Design review of the part built by this model. Coordinates are the model's own, in mm. Face numbers are marked on the shaded views. A direction names the side the tool comes from. Give positions to 0.01 mm unless a question says otherwise; leave off trailing zeros. Write each loop counter-clockwise with the first axis right and the second up, starting at its lowest first coordinate (ties: lowest second). Pieces come first, ordered by that corner, then holes. Notation, with made-up numbers: M 47.5,86 L 80.5,86 A17 cw 80.5,112 Z; hole C 20.5,68.5 d10. An arc over 180 degrees is marked long. Use one line per item in the form item = value. Start each with the question number.
from build123d import *

# Parameters (mm, degrees)
SKETCH1_R               = 25
BOSS_EXTRUDE1_DEPTH     = 10
SKETCH1_3_R             = 12.5
SKETCH1_3_R_2           = 6
BOSS_EXTRUDE2_DEPTH     = 35
CUT_EXTRUDE1_START      = 5
CUT_EXTRUDE1_DEPTH      = 5
CUT_EXTRUDE2_DEPTH      = 50.749371855
CUT_EXTRUDE2_DEPTH_BACK = 50.749371855
SKETCH3_R               = 2.5
CUT_EXTRUDE3_DEPTH      = 50.749371926
CIRPATTERN1_COUNT       = 6
CHAMFER1_SIZE           = 5


with BuildPart() as part:
    # Sketch1 → Boss-Extrude1 (new body)
    with BuildSketch(Plane(origin=(0, 0, 0), x_dir=(1, 0, 0), z_dir=(0, 1, 0))):
        with Locations(Location((0, 0, 0), (0, 0, 270))):
            Circle(SKETCH1_R)
    extrude(amount=BOSS_EXTRUDE1_DEPTH)

    # Sketch1<3> → Boss-Extrude2 (add)
    with BuildSketch(Plane(origin=(0, 0, 0), x_dir=(1, 0, 0), z_dir=(0, 1, 0))):
        with Locations(Location((0, 0, 0), (0, 0, 270))):
            Circle(SKETCH1_3_R)
        with Locations(Location((0, 0, 0), (0, 0, 270))):
            Circle(SKETCH1_3_R_2, mode=Mode.SUBTRACT)
    extrude(amount=BOSS_EXTRUDE2_DEPTH)

    # Sketch1<5> → Cut-Extrude1 (cut)
    with BuildSketch(Plane(origin=(0, 0, 0), x_dir=(1, 0, 0), z_dir=(0, 1, 0)).offset(CUT_EXTRUDE1_START)):
        with BuildLine():
            ThreePointArc((20, 15), (0, 25), (-20, 15))
            Line((-20, 15), (20, 15))
        make_face()
    extrude(amount=CUT_EXTRUDE1_DEPTH, mode=Mode.SUBTRACT)

    # Sketch2 → Cut-Extrude2 (cut, two sides: drawn at the far end of the back side and taken through both)
    with BuildSketch(Plane.XY.offset(-CUT_EXTRUDE2_DEPTH_BACK)):
        with BuildLine():
            Line((0, 25.5), (0, 35))
            Line((0, 35), (-2.5, 35))
            Line((-2.5, 35), (-2.5, 23))
            ThreePointArc((-2.5, 23), (-1.767766953, 24.767766953), (0, 25.5))
        make_face()
        with BuildLine():
            Line((2.5, 35), (0, 35))
            Line((0, 35), (0, 25.5))
            ThreePointArc((0, 25.5), (1.767766953, 24.767766953), (2.5, 23))
            Line((2.5, 23), (2.5, 35))
        make_face()
        with BuildLine():
            ThreePointArc((2.5, 23), (1.767766953, 24.767766953), (0, 25.5))
            Line((0, 25.5), (0, 23))
            Line((0, 23), (2.5, 23))
        make_face()
        with BuildLine():
            Line((0, 23), (0, 25.5))
            ThreePointArc((0, 25.5), (-1.767766953, 24.767766953), (-2.5, 23))
            Line((-2.5, 23), (0, 23))
        make_face()
        with BuildLine():
            Line((2.5, 23), (0, 23))
            Line((0, 23), (0, 20.5))
            ThreePointArc((0, 20.5), (1.767766953, 21.232233047), (2.5, 23))
        make_face()
        with BuildLine():
            Line((0, 20.5), (0, 23))
            Line((0, 23), (-2.5, 23))
            ThreePointArc((-2.5, 23), (-1.767766953, 21.232233047), (0, 20.5))
        make_face()
    extrude(amount=CUT_EXTRUDE2_DEPTH + CUT_EXTRUDE2_DEPTH_BACK, mode=Mode.SUBTRACT)

    # Sketch3 → Cut-Extrude3 (cut, through all)
    with BuildSketch(Plane(origin=(0, 0, 0), x_dir=(1, 0, 0), z_dir=(0, 1, 0))):
        with Locations(Location((0, 20, 0), (0, 0, 270))):
            Circle(SKETCH3_R)
    cut_extrude3 = extrude(amount=CUT_EXTRUDE3_DEPTH, mode=Mode.SUBTRACT)

    # CirPattern1: Cut-Extrude3 ×6 about axis
    cirpattern1_axis = Axis((0, 0, 0), (0, 1, 0))
    for i in range(1, CIRPATTERN1_COUNT):
        add(cut_extrude3.rotate(cirpattern1_axis, i * 360 / CIRPATTERN1_COUNT), mode=Mode.SUBTRACT)

    # Chamfer1
    chamfer1_edges = [part.edges().sort_by_distance(p)[0] for p in [
        (-12.5, 35, 0),
        (12.5, 35, 0),
    ]]
    chamfer(chamfer1_edges, length=CHAMFER1_SIZE)


solid = part.part
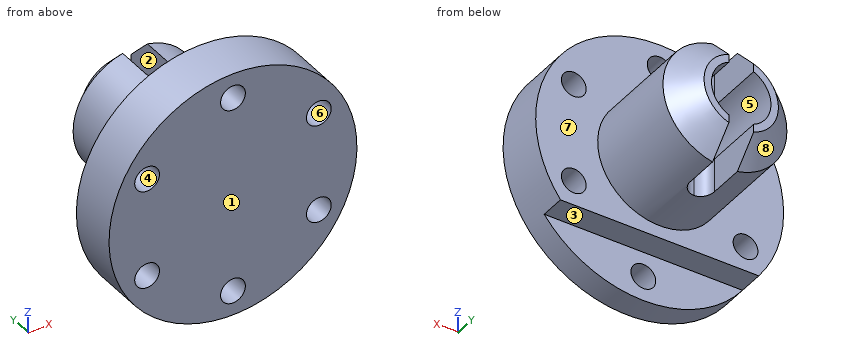
1. To check wall thickness, follow L1, parallel to Z at x = 0, y = 3; L2, parallel to X at y = 24.5, z = 0. State the ranges of each line that lie inside material, in increasing order.
2. For the marked faces 1, 2, 3, 4 and 5, list the 3-axis set-ups (+Z, -Z, +X, -X, +Y, -Y) from which the entire face can be reached by the end or side of a thin tool; tool diameter is ignored.
3. Clearance check with flat-ended pins moving along their axes: pin 1 Ø1 at (y, z) = (12.5, -6) entering from -X (3 decimals); pin 2 Ø6.5 at (x, z) = (-17.32, -10) entering from -Y; pin 3 Ø5.5 at (y, z) = (32, 8.5) entering from +X; pin 4 Ø3.5 at (y, z) = (28.5, -9.5) entering from +X. State where each tip first meets the part, or that it passes through.
4. Draft analysis for pull direction X (two halves, no side actions). For the marked faces 6, 7 and 8, state which applies: pulls with the +X half, pulls with the -X half, needs draft (parallel to the pull), parting line crosses it, or undercut.
5. We need section D-D (z = 0). State the section outline as (x, y) points.
6. We need section C-C (x = -16.5). State the section outline as (y, z) points, and give its area (3 significant figures).
7. We need section A-A (z = -20). State the section outline as (x, y) points.
8. We need section B-B (y = 29). State the section outline as (x, z) points, and give its area (3 significant figures).
Answer block:
q1.L1 = -25 to -22.5, -17.5 to 17.5, 22.5 to 25
q1.L2 = -12.5 to -6, 6 to 12.5
q2.face_1 = +Z, -Z, +X, -X, -Y
q2.face_2 = +Z, -Z, +Y
q2.face_3 = -Z, +X, -X, +Y
q2.face_4 = +Y, -Y
q2.face_5 = +Y
q3.pin_1 = -11.225
q3.pin_2 = 0
q3.pin_3 = 10.61
q3.pin_4 = 9.81
q4.face_6 = undercut
q4.face_7 = needs draft
q4.face_8 = pulls with the -X half
q5.outline = M -25,0 L 25,0 L 25,10 L 12.5,10 L 12.5,30 L 7.5,35 L 6,35 L 6,10 L -6,10 L -6,35 L -7.5,35 L -12.5,30 L -12.5,10 L -25,10 Z
q6.outline = M 0,-18.78 L 5,-18.78 L 5,-15 L 10,-15 L 10,-12.36 L 0,-12.36 Z; M 0,-7.64 L 10,-7.64 L 10,7.64 L 0,7.64 Z; M 0,12.36 L 10,12.36 L 10,18.78 L 0,18.78 Z
q6.area = 262 mm^2
q7.outline = M -15,0 L -2.5,0 L -2.5,5 L -15,5 Z; M 2.5,0 L 15,0 L 15,5 L 2.5,5 Z
q8.outline = M -2.5,-12.25 L -2.5,-5.45 A6 cw -2.5,5.45 L -2.5,12.25 A12.5 ccw Z; M 2.5,-12.25 A12.5 ccw 2.5,12.25 L 2.5,5.45 A6 cw 2.5,-5.45 Z
q8.area = 312 mm^2
